Design review of the part built by this model. Coordinates are the model's own, in mm. Coordinates: 2 decimals unless noted, no trailing zeros. Loops run counter-clockwise (first coordinate to the right, second up) from the corner with the lowest first, then second, coordinate; pieces in that order, holes last. Notation, with made-up numbers: (79, 47) -> (130, 47) arc R17 ccw to (130, 54) -> close; hole circle Ø9 at (47, -20). An arc over 180 degrees is marked (long way). Answer as a JSON object with one key per item and string values.
```python
from build123d import *

# Parameters (mm, degrees)
F1_DEPTH = 3.175
F2_R     = 3.17499


# Not quite as in the source:
# - a fillet or chamfer is up to 0.001 mm smaller than in the source, because OpenCascade refuses the exact size


with BuildPart() as f1:
    # F0 (on Right) → F1 (new body, symmetric)
    with BuildSketch(Plane.YZ):
        Polygon((3.175, 22.364773135), (0, 25.4), (-3.175, 22.364773135), (-5.08, 5.08), (-22.364773135, 3.175), (-25.4, 0), (-22.364773135, -3.175), (-5.08, -5.08), (-3.175, -22.364773135), (0, -25.4), (3.175, -22.364773135), (5.08, -5.08), (22.364773135, -3.175), (25.4, 0), (22.364773135, 3.175), (5.08, 5.08), align=None)
    extrude(amount=F1_DEPTH, both=True)

    # F2 (radius 3.175 in the source; OpenCascade refuses exactly that, so slightly less here)
    f2_edges = [f1.edges().sort_by_distance(p)[0] for p in [
        (3.175, 4.1275, 13.722387),
        (3.175, 1.5875, 23.882387),
        (3.175, -1.5875, 23.882387),
        (3.175, -4.1275, 13.722387),
        (3.175, -13.722387, 4.1275),
        (3.175, -23.882387, 1.5875),
        (3.175, -23.882387, -1.5875),
        (3.175, -13.722387, -4.1275),
        (3.175, -4.1275, -13.722387),
        (3.175, -1.5875, -23.882387),
        (3.175, 1.5875, -23.882387),
        (3.175, 4.1275, -13.722387),
        (3.175, 13.722387, -4.1275),
        (3.175, 23.882387, -1.5875),
        (3.175, 23.882387, 1.5875),
        (3.175, 13.722387, 4.1275),
        (-3.175, 4.1275, 13.722387),
        (-3.175, 1.5875, 23.882387),
        (-3.175, -1.5875, 23.882387),
        (-3.175, -4.1275, 13.722387),
        (-3.175, -13.722387, 4.1275),
        (-3.175, -23.882387, 1.5875),
        (-3.175, -23.882387, -1.5875),
        (-3.175, -13.722387, -4.1275),
        (-3.175, -4.1275, -13.722387),
        (-3.175, -1.5875, -23.882387),
        (-3.175, 1.5875, -23.882387),
        (-3.175, 4.1275, -13.722387),
        (-3.175, 13.722387, -4.1275),
        (-3.175, 23.882387, -1.5875),
        (-3.175, 23.882387, 1.5875),
        (-3.175, 13.722387, 4.1275),
    ]]
    fillet(f2_edges, radius=F2_R)


solid = f1.part
```
1) Clearance check with flat-ended pins moving along their axes: pin 1 Ø1.5 at (x, y) = (0.5, 16) entering from -Z; pin 2 Ø3 at (x, y) = (-0.5, 7.5) entering from -Z; pin 3 Ø1 at (x, z) = (2.5, -19) entering from +Y. State where each tip first meets the part, or that it passes through.
Completed:
{"pin 1": "z = -3.95", "pin 2": "z = -4.97", "pin 3": "y = 2.84"}
2) Add section A-A, the plane x = -1.5. Give the boundary of the cut face in (y, z).
Completed:
{"outline": "(-24.88, 0) -> (-22.19, -2.82) -> (-4.74, -4.74) -> (-2.82, -22.19) -> (0, -24.88) -> (2.82, -22.19) -> (4.74, -4.74) -> (22.19, -2.82) -> (24.88, 0) -> (22.19, 2.82) -> (4.74, 4.74) -> (2.82, 22.19) -> (0, 24.88) -> (-2.82, 22.19) -> (-4.74, 4.74) -> (-22.19, 2.82) -> close"}
3) Wall thickness on probe 1 along Y at (x, z) = (-2.5, 8); probe 2 along Y at (x, z) = (2, -5): over which ranges is each line inside the solid? List them lowest first.
Completed:
{"probe 1": "-3.53 to 3.53", "probe 2": "-4.38 to 4.38"}
4) Add section B-B, the plane x = 1.75. Give the boundary of the cut face in (y, z), and give its area (3 significant figures).
Completed:
{"outline": "(-24.67, 0) -> (-22.12, -2.67) -> (-4.6, -4.6) -> (-2.67, -22.12) -> (0, -24.67) -> (2.67, -22.12) -> (4.6, -4.6) -> (22.12, -2.67) -> (24.67, 0) -> (22.12, 2.67) -> (4.6, 4.6) -> (2.67, 22.12) -> (0, 24.67) -> (-2.67, 22.12) -> (-4.6, 4.6) -> (-22.12, 2.67) -> close", "area": "622 mm²"}
